```python
from build123d import *

# Parameters (mm, degrees)
F1_DEPTH        = 16
F2_W            = 12
F2_H            = 12
F4_DEPTH        = 15
F4_COPIES_COUNT = 8
F5_W            = 32
F5_H            = 32
F6_DEPTH        = 38.627


# Not quite as in the source:
# - a pattern or mirror of a feature is missing from the dataset's text; its kind, count and spacing are read off the source's solid


with BuildPart() as f1:
    # F0 (on Top) → F1 (new body, symmetric)
    with BuildSketch(Plane.XY):
        Polygon((-27.4452890516, 27.4452890516), (-38.8135, 0), (-27.4452890516, -27.4452890516), (0, -38.8135), (27.4452890516, -27.4452890516), (38.8135, 0), (27.4452890516, 27.4452890516), (0, 38.8135), align=None)
    extrude(amount=F1_DEPTH, both=True)

    # F2 (on face) → F4 (cut)
    with BuildSketch(Plane(origin=(-13.7226445258, -33.1293945258, 0), x_dir=(0.9238795325, -0.3826834324, 0), z_dir=(-0.3826834324, -0.9238795325, 0))):
        Rectangle(F2_W, F2_H)
    f4 = extrude(amount=-F4_DEPTH, mode=Mode.SUBTRACT)

    # F4_copies: F4 ×8 about axis
    f4_copies_axis = Axis((0, 0, 0), (0, 0, 1))
    for i in range(1, F4_COPIES_COUNT):
        add(f4.rotate(f4_copies_axis, i * 360 / F4_COPIES_COUNT), mode=Mode.SUBTRACT)


with BuildPart() as f6:
    # F5 (on Top) → F6 (new body, symmetric)
    with BuildSketch(Plane.XY):
        Rectangle(F5_W, F5_H)
    extrude(amount=F6_DEPTH, both=True)


solid = f1.part
```
Here's how the part is built. I have some questions about the finished solid (model axes, mm). A direction names the side the tool comes from. Coordinates: 2 decimals unless noted, no trailing zeros. Loops run counter-clockwise (first coordinate to the right, second up) from the corner with the lowest first, then second, coordinate; pieces in that order, holes last. Notation, with made-up numbers: M -23,88.5 L 27,88.5 A22 ccw 27,119.5 Z; hole C 18,11 d10. An arc over 180 degrees is marked long. One line per item, written item: value.
1. Thinking about a two-plate mould opening in Z: for faces 5 (the flat face through (-35.576, 7.816, 0.224)), 6 (the flat face through (-5.35, 28.59, -0.08)), which applies, +Z half, -Z half, draft (parallel to the pull), parting line (faces both ways), or undercut?
Geometry says:
face 5: draft
face 6: undercut
2. Imagine slicing it at B-B (z = -9.5). List the corners of the cut face in (x, y) for me.
Geometry says:
outline: M -38.81,0 L -27.45,-27.45 L 0,-38.81 L 27.45,-27.45 L 38.81,0 L 27.45,27.45 L 0,38.81 L -27.45,27.45 Z
3. Please list where these lines run through material, in increasing order: probe 1 along Z at (x, y) = (-25.5, -5.5); probe 2 along Y at (x, z) = (-3, -0.5); probe 3 along X at (y, z) = (18.5, -0.5).
Geometry says:
probe 1: z = -16 to -6, 6 to 16
probe 2: y = -37.57 to -22.92, -21.33 to 21.33, 22.92 to 37.57
probe 3: x = -28.98 to -14.16, -9.84 to 9.84, 14.16 to 28.98
4. Will these pins go through, and if not, where does the flat tip stop? pin 1 Ø1 at (x, z) = (5.5, 1) entering from +Y; pin 2 Ø3 at (y, z) = (-27, 9.5) entering from +X; pin 3 Ø10 at (y, z) = (25.5, -12) entering from +X.
Geometry says:
pin 1: stops at y = 36.74
pin 2: stops at x = 28.25
pin 3: stops at x = 30.32
5. On a 3-axis mill with a long thin cutter (end or side, diameter ignored), from which of +Z, -Z, +X, -X, +Y, -Y can I reach the whole of each face in a straight line? I mean faces 1 (the flat face through (26, -11, 6)), 2 (the flat face through (-24.001, -16.436, -0.084)), 3 (the flat face through (-16.436, -24.001, -0.084)), 4 (the flat face through (24.001, -16.436, -0.084)). Say none if no direction works.
Geometry says:
face 1: none
face 2: -X
face 3: -Y
face 4: +X
6. Imagine slicing it at D-D (y = -18). List the corners of the cut face in (x, z) for me, and give its area (3 significant figures).
Geometry says:
outline: M -31.36,-16 L 31.36,-16 L 31.36,-6 L 27.78,-6 L 27.78,6 L 31.36,6 L 31.36,16 L -31.36,16 L -31.36,6 L -27.78,6 L -27.78,-6 L -31.36,-6 Z; hole M -13.95,-6 L -11.05,-6 L -11.05,6 L -13.95,6 Z; hole M 11.05,-6 L 13.95,-6 L 13.95,6 L 11.05,6 Z
area: 1,850 mm2
7. Imagine slicing it at A-A (x = -26). List the corners of the cut face in (y, z) for me, and give its area (3 significant figures).
Geometry says:
outline: M -28.04,-16 L 28.04,-16 L 28.04,16 L -28.04,16 Z; hole M -17.26,-6 L -4.28,-6 L -4.28,6 L -17.26,6 Z; hole M 4.28,-6 L 17.26,-6 L 17.26,6 L 4.28,6 Z
area: 1,480 mm2
8. Imagine slicing it at C-C (y = 15). List the corners of the cut face in (x, z) for me.
Geometry says:
outline: M -32.6,-16 L 32.6,-16 L 32.6,-6 L 20.53,-6 L 20.53,6 L 32.6,6 L 32.6,16 L -32.6,16 L -32.6,6 L -20.53,6 L -20.53,-6 L -32.6,-6 Z
